```python
from build123d import *

# Parameters (mm, degrees)
F0_R     = 7.825
F0_R_2   = 3.5
F1_DEPTH = 6.03
F0_R_3   = 2.45
F2_DEPTH = 2.68
F3_R     = 6.65919
F3_R_2   = 4.726229
F4_DEPTH = 2


with BuildPart() as f1:
    # F0 (on Top) → F1 (new body)
    with BuildSketch(Plane.XY):
        Circle(F0_R)
        Circle(F0_R_2, mode=Mode.SUBTRACT)
    extrude(amount=F1_DEPTH)

    # F0 (on Top) → F2 (join)
    with BuildSketch(Plane.XY):
        Circle(F0_R_2)
        Circle(F0_R_3, mode=Mode.SUBTRACT)
    extrude(amount=F2_DEPTH)

    # F3 (on face) → F4 (cut)
    with BuildSketch(Plane.XY.offset(6.03)):
        Circle(F3_R)
        Circle(F3_R_2, mode=Mode.SUBTRACT)
    extrude(amount=-F4_DEPTH, mode=Mode.SUBTRACT)


solid = f1.part
```
Geometry: final body of the model. Coordinates: model frame, mm. A direction names the side the tool comes from. Give positions to 0.01 mm unless a question says otherwise; leave off trailing zeros. Loops run counter-clockwise (first coordinate to the right, second up) from the corner with the lowest first, then second, coordinate; pieces in that order, holes last. Notation, with made-up numbers: (1.5, -4) -> (47.5, -4) arc R14 ccw to (47.5, 14) -> close; hole circle Ø8 at (65.5, -34). An arc over 180 degrees is marked (long way). Use one line per item in the form item = value.
Item 1: Pin query (flat end, axial travel): P1, Ø2, axis at y = 2, z = 4, coming from the +X side; P2, Ø1.5, axis at y = 2, z = 3.5, coming from the +X side; P3, Ø1.5, axis at x = 3, z = 4, coming from the +Y side. Return the tip coordinate at first contact, or that it passes through.
A:
P1 = 7.76
P2 = 7.72
P3 = 7.49
Item 2: Section query A-A on x = 0. Output: boundary loops of the cut face in (y, z) (3 decimals).
A:
outline = (-7.825, 0) -> (-2.45, 0) -> (-2.45, 2.68) -> (-3.5, 2.68) -> (-3.5, 6.03) -> (-4.726, 6.03) -> (-4.726, 4.03) -> (-6.659, 4.03) -> (-6.659, 6.03) -> (-7.825, 6.03) -> close; (2.45, 0) -> (7.825, 0) -> (7.825, 6.03) -> (6.659, 6.03) -> (6.659, 4.03) -> (4.726, 4.03) -> (4.726, 6.03) -> (3.5, 6.03) -> (3.5, 2.68) -> (2.45, 2.68) -> close
Item 3: Line query: probe 1 along Y at (x, z) = (0, 5.35) (3 decimals); probe 2 along X at (y, z) = (-2.5, 4.75); probe 3 along Y at (x, z) = (0, 1.2) (3 decimals). Output: solid intervals per line, ascending.
A:
probe_1 = -7.825 to -6.659, -4.726 to -3.5, 3.5 to 4.726, 6.659 to 7.825
probe_2 = -7.41 to -6.17, -4.01 to -2.45, 2.45 to 4.01, 6.17 to 7.41
probe_3 = -7.825 to -2.45, 2.45 to 7.825
Item 4: Access query for faces 4 (the face through (4.508, 1.42, 5.044)), 5 (the face through (-0.5, -2.4, 1.3)). Directions: +Z, -Z, +X, -X, +Y, -Y. A direction counts if a zero-diameter tool reaches every point of the face in a straight line with its end or side. Return the directions, or none.
A:
face_4 = +Z
face_5 = +Z, -Z
Item 5: Section query D-D on x = -6.25. Output: boundary loops of the cut face in (y, z).
A:
outline = (-4.71, 0) -> (4.71, 0) -> (4.71, 6.03) -> (2.3, 6.03) -> (2.3, 4.03) -> (-2.3, 4.03) -> (-2.3, 6.03) -> (-4.71, 6.03) -> close
Item 6: Draft query along Y for faces 1 (the face through (2, 2, 0)), 2 (the face through (-1.02, 7.76, 2.97)), 3 (the face through (1, 5, 4.03)). Return one class per face: pulls with the +Y half, pulls with the -Y half, needs draft (parallel to the pull), parting line crosses it, or undercut.
A:
face_1 = needs draft
face_2 = parting line crosses it
face_3 = undercut
Item 7: Section query C-C on z = 5.25. Output: boundary loops of the cut face in (x, y) (3 decimals), and give its area (3 significant figures).
A:
outline = circle Ø15.65 at (0, 0); circle Ø9.452 at (0, 0); hole circle Ø13.318 at (0, 0); hole circle Ø7 at (0, 0)
area = 84.7 mm^2
